```python
from build123d import *

# Parameters (mm, degrees)
SKETCH_1_R      = 3.25
SKETCH_1_R_2    = 7.5
EXTRUDE_1_DEPTH = 1
SKETCH_2_R      = 6.75
SKETCH_2_R_2    = 2.75
EXTRUDE_2_DEPTH = 2.5
CHAMFER_1_SIZE  = 0.8
SKETCH_3_R      = 1
EXTRUDE_3_DEPTH = 0.55


with BuildPart() as part:
    # 草图1 → 凸台-拉伸1 (new body)
    with BuildSketch(Plane(origin=(0, 0, 0), x_dir=(1, 0, 0), z_dir=(0, 1, 0))):
        with Locations((-4.465418824, 10.828840308)):
            Circle(SKETCH_1_R)
        with BuildLine():
            Line((-3.953247825, 7.619450823), (-3.538203787, 6.612950473))
            ThreePointArc((-3.538203787, 6.612950473), (-2.859173271, 6.933623022), (-2.151479183, 7.184785127))
            Line((-2.151479183, 7.184785127), (-2.56652322, 8.191285477))
            ThreePointArc((-2.56652322, 8.191285477), (-3.22644374, 7.824270332), (-3.953247825, 7.619450823))
        make_face()
        Circle(SKETCH_1_R_2)
        with Locations((4.416088752, 11.919352316)):
            Circle(SKETCH_1_R)
        with BuildLine():
            Line((2.404044607, 9.367063468), (1.64466801, 7.317449497))
            ThreePointArc((1.64466801, 7.317449497), (2.605643113, 7.03282475), (3.520087943, 6.622611333))
            Line((3.520087943, 6.622611333), (4.279464541, 8.672225305))
            ThreePointArc((4.279464541, 8.672225305), (3.286976736, 8.871794924), (2.404044607, 9.367063468))
        make_face()
        with BuildLine():
            ThreePointArc((6.059916763, 4.418982782), (6.595006984, 3.571537887), (7.012326866, 2.660314252))
            Line((7.012326866, 2.660314252), (8.926399669, 3.696883819))
            ThreePointArc((8.926399669, 3.696883819), (8.311549297, 4.501134462), (7.973989566, 5.455552349))
            Line((7.973989566, 5.455552349), (6.059916763, 4.418982782))
        make_face()
        with Locations((11.169385657, 6.048800879)):
            Circle(SKETCH_1_R)
        with Locations((11.325553388, -2.898042413)):
            Circle(SKETCH_1_R)
        with BuildLine():
            Line((7.043551493, -2.576505845), (8.076059132, -2.840709353))
            ThreePointArc((8.076059132, -2.840709353), (8.176998527, -2.092373567), (8.447906292, -1.387530186))
            Line((8.447906292, -1.387530186), (7.415398652, -1.123326679))
            ThreePointArc((7.415398652, -1.123326679), (7.265895832, -1.859235798), (7.043551493, -2.576505845))
        make_face()
    extrude(amount=EXTRUDE_1_DEPTH)

    # 草图2 → 凸台-拉伸2 (add)
    with BuildSketch(Plane(origin=(0, 1, 0), x_dir=(1, 0, 0), z_dir=(0, 1, 0))):
        with Locations(Location((0, 0, 0), (0, 0, 270))):
            Circle(SKETCH_2_R)
        with Locations(Location((-4.465418824, 10.828840308, 0), (0, 0, 270))):
            Circle(SKETCH_2_R_2)
        with Locations(Location((4.416088752, 11.919352316, 0), (0, 0, 270))):
            Circle(SKETCH_2_R_2)
        with Locations(Location((11.169385657, 6.048800879, 0), (0, 0, 270))):
            Circle(SKETCH_2_R_2)
        with Locations(Location((11.325553388, -2.898042413, 0), (0, 0, 270))):
            Circle(SKETCH_2_R_2)
    extrude(amount=EXTRUDE_2_DEPTH)

    # 倒角1
    chamfer_1_edges = [part.edges().sort_by_distance(p)[0] for p in [
        (0, 3.5, -6.75),
        (-4.465418824, 3.5, -13.578840308),
        (4.416088752, 3.5, -14.669352316),
        (11.169385657, 3.5, -8.798800879),
        (11.325553388, 3.5, 0.148042413),
    ]]
    chamfer(chamfer_1_edges, length=CHAMFER_1_SIZE)

    # 草图3 → 凸台-拉伸3 (add)
    with BuildSketch(Plane.XZ):
        with Locations(Location((0, 0, 0), (0, 0, 90))):
            Circle(SKETCH_3_R)
        with Locations(Location((11.325553388, 2.898042413, 0), (0, 0, 90))):
            Circle(SKETCH_3_R)
        with Locations(Location((11.169385657, -6.048800879, 0), (0, 0, 90))):
            Circle(SKETCH_3_R)
        with Locations(Location((4.416088752, -11.919352316, 0), (0, 0, 90))):
            Circle(SKETCH_3_R)
        with Locations(Location((-4.465418824, -10.828840308, 0), (0, 0, 90))):
            Circle(SKETCH_3_R)
    extrude(amount=EXTRUDE_3_DEPTH)


solid = part.part
```
CAD build for the part. Positions are in the model's coordinates, mm. A direction names the side the tool comes from. Round coordinates to 2 decimals unless told otherwise and drop trailing zeros. Write each loop counter-clockwise with the first axis right and the second up, starting at its lowest first coordinate (ties: lowest second). Pieces come first, ordered by that corner, then holes. Notation, with made-up numbers: (41.25, -7.5) -> (74.25, -7.5) arc R15 ccw to (74.25, 16.5) -> close; hole circle Ø4 at (-12, 46.25). An arc over 180 degrees is marked (long way). Answer in a Markdown table with one row per item. Add a question column.
Item 1: Saw through at B-B, the plane x = 0. Write the cut outline in (y, z).
Item 2: Drill centre lines: line 1 (Y direction, x = 7.75, z = -4.5); line 2 (X direction, y = 1.2, z = -4.5); line 3 (Z direction, x = -5, y = 1.8). Where is each one in solid material? Low to high. Write a range as from..to.
Item 3: Saw through at A-A, the plane y = 1.4. Write the cut outline in (x, z), then the cut area to 3 significant figures.
Item 4: Mould opens along X. For faces 6 (the face through (-4, 3.5, -11)), 7 (the face through (7.553, 0.493, 2.707)), 8 (the face through (11.13, -0.27, -7.05)) say: pulls with the +X half, pulls with the -X half, needs draft (parallel to the pull), parting line crosses it, or undercut.
Item 5: Which spindle directions (+Z, -Z, +X, -X, +Y, -Y) get a long thin tool onto all of the face, cutting with end or side? Do faces 1 (the face through (-0.235, 0.493, -7.496)), 2 (the face through (0, 3.5, 0)), 3 (the face through (8.73, 1.84, -4.78)), 4 (the face through (0, -0.55, 0)), 5 (the face through (0.976, -0.271, -0.217)). Say none if no direction does.
Item 6: Drop a flat-ended pin along its axis: pin 1 Ø1 at (x, y) = (4.5, 2) entering from -Z. Give the stop position or say it passes through.
Item 7: Saw through at C-C, the plane y = 3.1. Write the cut outline in (x, z), then the cut area to 3 significant figures.
Findings below:
| question | item | result |
|---|---|---|
| 1 | outline | (-0.55, -1) -> (0, -1) -> (0, -7.5) -> (1, -7.5) -> (1, -6.75) -> (2.7, -6.75) -> (3.5, -5.95) -> (3.5, 5.95) -> (2.7, 6.75) -> (1, 6.75) -> (1, 7.5) -> (0, 7.5) -> (0, 1) -> (-0.55, 1) -> close |
| 2 | line 1 | y = 0..1 |
| 2 | line 2 | x = -5.03..5.03, 8.9..13.44 |
| 2 | line 3 | z = -13.53..-8.13, -4.53..4.53 |
| 3 | outline | circle Ø5.5 at (-4.47, -10.83); circle Ø13.5 at (0, 0); circle Ø5.5 at (4.42, -11.92); circle Ø5.5 at (11.17, -6.05); circle Ø5.5 at (11.33, 2.9) |
| 3 | area | 238 mm^2 |
| 4 | face 6 | needs draft |
| 4 | face 7 | undercut |
| 4 | face 8 | parting line crosses it |
| 5 | face 1 | +Y, -Y |
| 5 | face 2 | +Z, -Z, +X, -X, +Y |
| 5 | face 3 | +Y |
| 5 | face 4 | +Z, -Z, +X, -X, -Y |
| 5 | face 5 | -Y |
| 6 | pin 1 | stops at z = -14.67 |
| 7 | outline | circle Ø4.7 at (-4.47, -10.83); circle Ø12.7 at (0, 0); circle Ø4.7 at (4.42, -11.92); circle Ø4.7 at (11.17, -6.05); circle Ø4.7 at (11.33, 2.9) |
| 7 | area | 196 mm^2 |
